from build123d import *

# Parameters (mm, degrees)
SKETCH_1_R          = 26
EXTRUDE_1_DEPTH     = 4
SKETCH_2_R          = 18
EXTRUDE_2_DEPTH     = 20.5
SKETCH_3_R          = 13
CUT_EXTRUDE_1_DEPTH = 11.5
SKETCH_4_R          = 2.2
CUT_EXTRUDE_2_DEPTH = 1
SKETCH_5_R          = 1.1
CUT_EXTRUDE_3_DEPTH = 43.09809972
SKETCH_6_R          = 11
CUT_EXTRUDE_4_DEPTH = 40
SKETCH_7_R          = 1
CUT_EXTRUDE_5_DEPTH = 5


with BuildPart() as part:
    # Эскиз1 → Бобышка-Вытянуть1 (new body)
    with BuildSketch(Plane(origin=(0, 0, 0), x_dir=(1, 0, 0), z_dir=(0, 1, 0))):
        with Locations(Location((0, 0, 0), (0, 0, 270))):
            Circle(SKETCH_1_R)
    extrude(amount=EXTRUDE_1_DEPTH)

    # Эскиз2 → Бобышка-Вытянуть2 (add)
    with BuildSketch(Plane(origin=(0, 4, 0), x_dir=(1, 0, 0), z_dir=(0, 1, 0))):
        with Locations(Location((0, 0, 0), (0, 0, 270))):
            Circle(SKETCH_2_R)
    extrude(amount=EXTRUDE_2_DEPTH)

    # Эскиз3 → Вырез-Вытянуть1 (cut)
    with BuildSketch(Plane(origin=(0, 24.5, 0), x_dir=(1, 0, 0), z_dir=(0, 1, 0))):
        with Locations(Location((0, 0, 0), (0, 0, 270))):
            Circle(SKETCH_3_R)
    extrude(amount=-CUT_EXTRUDE_1_DEPTH, mode=Mode.SUBTRACT)

    # Эскиз4 → Вырез-Вытянуть2 (cut)
    with BuildSketch(Plane(origin=(0, 4, 0), x_dir=(1, 0, 0), z_dir=(0, 1, 0))):
        with Locations(Location((-22, 0, 0), (0, 0, 270))):
            Circle(SKETCH_4_R)
        with Locations(Location((0, 22, 0), (0, 0, 270))):
            Circle(SKETCH_4_R)
        with Locations(Location((22, 0, 0), (0, 0, 270))):
            Circle(SKETCH_4_R)
        with Locations(Location((0, -22, 0), (0, 0, 270))):
            Circle(SKETCH_4_R)
    extrude(amount=-CUT_EXTRUDE_2_DEPTH, mode=Mode.SUBTRACT)

    # Эскиз5 → Вырез-Вытянуть3 (cut, through all)
    with BuildSketch(Plane(origin=(0, 4, 0), x_dir=(1, 0, 0), z_dir=(0, 1, 0))):
        with Locations(Location((-22, 0, 0), (0, 0, 270))):
            Circle(SKETCH_5_R)
        with Locations(Location((0, 22, 0), (0, 0, 270))):
            Circle(SKETCH_5_R)
        with Locations(Location((22, 0, 0), (0, 0, 270))):
            Circle(SKETCH_5_R)
        with Locations(Location((0, -22, 0), (0, 0, 270))):
            Circle(SKETCH_5_R)
    extrude(amount=-CUT_EXTRUDE_3_DEPTH, mode=Mode.SUBTRACT)

    # Эскиз6 → Вырез-Вытянуть4 (cut, through all)
    with BuildSketch(Plane(origin=(0, 13, 0), x_dir=(1, 0, 0), z_dir=(0, 1, 0))):
        with Locations(Location((0, 0, 0), (0, 0, 270))):
            Circle(SKETCH_6_R)
    extrude(amount=-CUT_EXTRUDE_4_DEPTH, mode=Mode.SUBTRACT)

    # Эскиз7 → Вырез-Вытянуть5 (cut)
    with BuildSketch(Plane(origin=(0, 24.5, 0), x_dir=(1, 0, 0), z_dir=(0, 1, 0))):
        with Locations(Location((-15.5, 0, 0), (0, 0, 270))):
            Circle(SKETCH_7_R)
        with Locations(Location((0, 15.5, 0), (0, 0, 270))):
            Circle(SKETCH_7_R)
        with Locations(Location((15.5, 0, 0), (0, 0, 270))):
            Circle(SKETCH_7_R)
        with Locations(Location((0, -15.5, 0), (0, 0, 270))):
            Circle(SKETCH_7_R)
    extrude(amount=-CUT_EXTRUDE_5_DEPTH, mode=Mode.SUBTRACT)


solid = part.part
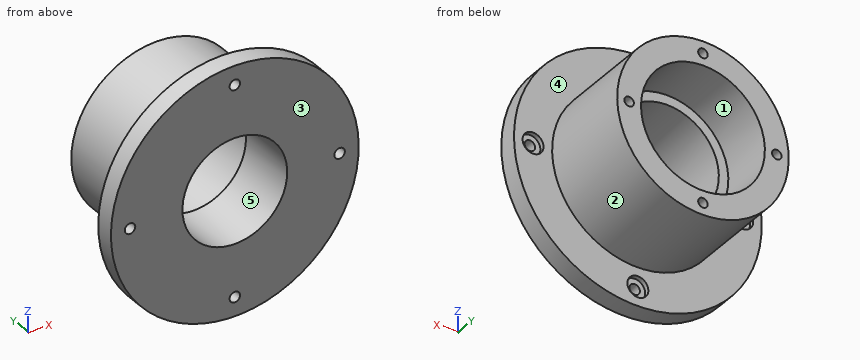
For this review, take the finished solid that the model builds, in its own axes (mm). Face numbers are marked on the shaded views. A direction names the side the tool comes from. Coordinates: 2 decimals unless noted, no trailing zeros. Order: outer loops, then holes, each group sorted by start corner. A loop starts at its lowest first (then second) coordinate and runs counter-clockwise, first axis right, second up. Notation, with made-up numbers: (88, 25) - (107, 25) arc R29 ccw to (107, 54) - close; hole circle Ø10 at (43.5, 56). An arc over 180 degrees is marked (long way). Answer as CSV lines item,"result". Start each with the question number.
1) Add section A-A (z = -22). State the section outline as (x, y) points.
2) Machinability: for the marked faces 4 and 5, which of the approach directions +Z, -Z, +X, -X, +Y, -Y give a long, thin tool a straight path to every point of the face, cutting with its end or side? Answer none if there is none.
3) Insertion check: P1, Ø5, axis at x = -1, z = -21, coming from the +Y side; P2, Ø4, axis at x = 22, z = 0, coming from the +Y side; P3, Ø2.5, axis at x = 15.5, z = 0, coming from the +Y side; P4, Ø1.5, axis at x = 20.5, y = 4.5, coming from the +Z side. Each pin has a flat end and moves straight along its axis. Give the tip position at first contact, or say it passes through.
4) Add section C-C (y = 11.5). State the section outline as (x, z) points.
5) To check wall thickness, follow line 1 along X through (y, z) = (3.65, 0); line 2 along X through (y, z) = (22.8, 0); line 3 along X through (y, z) = (19.25, 0). State the ranges of each line that lie inside material, in increasing order. Write a range as [from, to].
6) Add section B-B (x = 22). State the section outline as (y, z) points, then the cut area to 3 significant figures.
7) Add section D-D (z = 0). Count the separate pieces of the cut face and the enclosed holes in it, then the cut area to 3 significant figures.
8) Draft analysis for pull direction X (two halves, no side actions). For the marked faces 1, 2 and 3, state which applies: +X half, -X half, draft (parallel to the pull), parting line (faces both ways), or undercut.
Result:
1,outline,"(-13.86, 0) - (-1.1, 0) - (-1.1, 3) - (-2.2, 3) - (-2.2, 4) - (-13.86, 4) - close; (1.1, 0) - (13.86, 0) - (13.86, 4) - (2.2, 4) - (2.2, 3) - (1.1, 3) - close"
2,face 4,"+Y"
2,face 5,"+Y, -Y"
3,P1,"y = 4"
3,P2,"y = 3"
3,P3,"y = 24.5"
3,P4,"z = 16.68"
4,outline,"circle Ø36 at (0, 0); hole circle Ø22 at (0, 0)"
5,line 1,"[-26, -24.2], [-19.8, -11], [11, 19.8], [24.2, 26]"
5,line 2,"[-18, -16.5], [-14.5, -13], [13, 14.5], [16.5, 18]"
5,line 3,"[-18, -13], [13, 18]"
6,outline,"(0, -13.86) - (4, -13.86) - (4, -2.2) - (3, -2.2) - (3, -1.1) - (0, -1.1) - close; (0, 1.1) - (3, 1.1) - (3, 2.2) - (4, 2.2) - (4, 13.86) - (0, 13.86) - close"
6,area,"99.9 mm^2"
7,separate pieces,"4"
7,enclosed holes,"0"
7,area,"319 mm^2"
8,face 1,"undercut"
8,face 2,"parting line"
8,face 3,"draft"
